Autodesk Inventor part; units mm, degrees
ref_plane "YZ Plane" through (0, 0, 0) normal (1, 0, 0) x (0, 1, 0)
ref_plane "XZ Plane" through (0, 0, 0) normal (0, 1, 0) x (-1, 0, 0)
ref_plane "XY Plane" through (0, 0, 0) normal (0, 0, 1) x (1, 0, 0)
sketch "스케치1" plane through (0, 0, 0) normal (0, 0, 1) x (1, 0, 0)
  line L0 (0, 0) -> (20, 0)
  line L1 (20, 0) -> (20, -20)
  line L2 (20, -20) -> (0, -20)
  line L3 (0, -20) -> (0, 0)
  line L4 (-2, 2) -> (21, 2)
  line L5 (21, 2) -> (21, -22)
  line L6 (21, -22) -> (-2, -22)
  line L7 (-2, -22) -> (-2, 2)
  line L8 (21, 2) -> (21, 5)
  line L9 (21, 5) -> (46, 5)
  line L10 (46, 5) -> (46, -22)
  line L11 (46, -22) -> (21, -22)
  line L12 (22, 3) -> (45, 3)
  line L13 (45, 3) -> (45, -20)
  line L14 (45, -20) -> (22, -20)
  line L15 (22, -20) -> (22, 3)
  line L16 (46, 5) -> (46, 8)
  line L17 (46, 8) -> (74, 8)
  line L18 (74, 8) -> (74, -22)
  line L19 (74, -22) -> (46, -22)
  line L20 (47, 6) -> (73, 6)
  line L21 (73, 6) -> (73, -20)
  line L22 (73, -20) -> (47, -20)
  line L23 (47, -20) -> (47, 6)
  line L24 (74, 8) -> (74, 11)
  line L25 (74, 11) -> (105, 11)
  line L26 (105, 11) -> (105, -22)
  line L27 (105, -22) -> (74, -22)
  line L28 (75, 9) -> (104, 9)
  line L29 (104, 9) -> (104, -20)
  line L30 (104, -20) -> (75, -20)
  line L31 (75, -20) -> (75, 9)
  line L32 (105, 11) -> (105, 14)
  line L33 (105, 14) -> (139, 14)
  line L34 (139, 14) -> (139, -22)
  line L35 (139, -22) -> (105, -22)
  line L36 (106, 12) -> (138, 12)
  line L37 (138, 12) -> (138, -20)
  line L38 (138, -20) -> (106, -20)
  line L39 (106, -20) -> (106, 12)
  line L40 (139, 14) -> (139, 17)
  line L41 (139, 17) -> (177, 17)
  line L42 (177, 17) -> (177, -22)
  line L43 (177, -22) -> (139, -22)
  line L44 (140, 15) -> (175, 15)
  line L45 (175, 15) -> (175, -20)
  line L46 (175, -20) -> (140, -20)
  line L47 (140, -20) -> (140, 15)
  dimension "d0" = 20
  dimension "d1" = 20
  dimension "d2" = 2
  dimension "d3" = 2
  dimension "d4" = 1
  dimension "d5" = 2
  dimension "d6" = 25
  dimension "d7" = 27
  dimension "d8" = 1
  dimension "d9" = 2
  dimension "d10" = 2
  dimension "d11" = 1
  dimension "d12" = 30
  dimension "d13" = 28
  dimension "d14" = 2
  dimension "d15" = 1
  dimension "d16" = 1
  dimension "d17" = 2
  dimension "d18" = 31
  dimension "d19" = 33
  dimension "d20" = 2
  dimension "d21" = 2
  dimension "d22" = 1
  dimension "d23" = 1
  dimension "d24" = 34
  dimension "d25" = 36
  dimension "d26" = 2
  dimension "d27" = 1
  dimension "d28" = 2
  dimension "d29" = 1
  dimension "d30" = 38
  dimension "d31" = 39
  dimension "d32" = 2
  dimension "d33" = 1
  dimension "d34" = 2
  dimension "d35" = 2
extrude "돌출1" add sketch "스케치1" along normal blind 4
sketch "스케치2" plane through (0, 0, 4) normal (0, 0, 1) x (1, 0, 0)
  line L0 (-2, -22) -> (177, -22)
  line L1 (177, -22) -> (177, 17)
  line L2 (177, 17) -> (139, 17)
  line L3 (139, 17) -> (139, 14)
  line L4 (139, 14) -> (105, 14)
  line L5 (105, 14) -> (105, 11)
  line L6 (105, 11) -> (74, 11)
  line L7 (74, 11) -> (74, 8)
  line L8 (74, 8) -> (46, 8)
  line L9 (46, 8) -> (46, 5)
  line L10 (46, 5) -> (21, 5)
  line L11 (21, 5) -> (21, 2)
  line L12 (21, 2) -> (-2, 2)
  line L13 (-2, 2) -> (-2, -22)
  line L14 (22, 3) -> (45, 3)
  line L15 (45, 3) -> (45, -20)
  line L16 (45, -20) -> (22, -20)
  line L17 (22, -20) -> (22, 3)
  line L18 (47, 6) -> (73, 6)
  line L19 (73, 6) -> (73, -20)
  line L20 (73, -20) -> (47, -20)
  line L21 (47, -20) -> (47, 6)
  line L22 (75, 9) -> (104, 9)
  line L23 (104, 9) -> (104, -20)
  line L24 (104, -20) -> (75, -20)
  line L25 (75, -20) -> (75, 9)
  line L26 (106, 12) -> (138, 12)
  line L27 (138, 12) -> (138, -20)
  line L28 (138, -20) -> (106, -20)
  line L29 (106, -20) -> (106, 12)
  line L30 (140, 15) -> (175, 15)
  line L31 (175, 15) -> (175, -20)
  line L32 (175, -20) -> (140, -20)
  line L33 (140, -20) -> (140, 15)
  line L34 (0, 0) -> (20, 0)
  line L35 (20, 0) -> (20, -20)
  line L36 (20, -20) -> (0, -20)
  line L37 (0, -20) -> (0, 0)
extrude "돌출2" add sketch "스케치2" along normal blind 1 contours L13 L12 L11 L10 L9 L8 L7 L6 L5 L4 L3 L2 L1 L0 | L14 L15 L16 L17 | L18 L19 L20 L21 | L22 L23 L24 L25 | L26 L27 L28 L29 | L30 L31 L32 L33 | L34 L35 L36 L37
fillet "모깎기1" radius 2 9 edges at (177, -22, 2.5) (177, 17, 2.5) (139, 17, 2.5) (105, 14, 2.5) (74, 11, 2.5) (46, 8, 2.5) (21, 5, 2.5) (-2, 2, 2.5) (-2, -22, 2.5)
properties part number "d_pocket"
Here's how the part is built. I have some questions about the finished solid (model axes, mm). A direction names the side the tool comes from. Coordinates: 2 decimals unless noted, no trailing zeros. Order: outer loops, then holes, each group sorted by start corner. A loop starts at its lowest first (then second) coordinate and runs counter-clockwise, first axis right, second up.
Item 1: If we section it at A-A, the plane x = 125.5: List the corners of the cut face in (y, z) for me.
Response values:
outline: (-22, 0) - (-20, 0) - (-20, 4) - (12, 4) - (12, 0) - (14, 0) - (14, 5) - (-22, 5) - close
Item 2: I need wall thicknesses on probe 1 along Y at (x, z) = (29.5, 3.35); probe 2 along Y at (x, z) = (81, 1.5); probe 3 along X at (y, z) = (0.5, 2.95). Which ranges of each line are inside material? Lowest first, please.
Response values:
probe 1: y = -22 to -20, 3 to 5
probe 2: y = -22 to -20, 9 to 11
probe 3: x = -1.94 to 22, 45 to 47, 73 to 75, 104 to 106, 138 to 140, 175 to 177
Item 3: If we section it at C-C, the plane z = 0.9: Give the number of separate pieces and of enclosed holes in the cut face, then the cut area to 3 significant figures.
Response values:
separate pieces: 1
enclosed holes: 6
area: 1,090 mm2
Item 4: If we section it at B-B, the plane y = -7: List the corners of the cut face in (x, z) for me.
Response values:
outline: (-2, 0) - (0, 0) - (0, 4) - (20, 4) - (20, 0) - (22, 0) - (22, 4) - (45, 4) - (45, 0) - (47, 0) - (47, 4) - (73, 4) - (73, 0) - (75, 0) - (75, 4) - (104, 4) - (104, 0) - (106, 0) - (106, 4) - (138, 4) - (138, 0) - (140, 0) - (140, 4) - (175, 4) - (175, 0) - (177, 0) - (177, 5) - (-2, 5) - close
Item 5: If we section it at D-D, the plane x = 102.5: List the corners of the cut face in (y, z) for me.
Response values:
outline: (-22, 0) - (-20, 0) - (-20, 4) - (9, 4) - (9, 0) - (11, 0) - (11, 5) - (-22, 5) - close
Item 6: I'm going to push flat-ended pins straight in: pin 1 Ø1.2 at (x, z) = (55, 1) entering from +Y; pin 2 Ø2 at (x, z) = (103, 0.5) entering from +Y; pin 3 Ø6 at (x, y) = (143.5, 2.5) entering from -Z. Where does each tip first touch, or does it pass through?
Response values:
pin 1: stops at y = 8
pin 2: stops at y = 11
pin 3: stops at z = 4
Item 7: Which directions (+Z, -Z, +X, -X, +Y, -Y) give clear straight access to the entire face, cutting with the end or side of a thin tool? Please do faces 4 (the face through (158, -20, 2)), 5 (the face through (10, 2, 2)).
Response values:
face 4: -Z
face 5: +Z, -Z, -X, +Y
Item 8: Thinking about a two-plate mould opening in Y: for faces 1 (the face through (90, 11, 2)), 2 (the face through (122, -20, 2)), 3 (the face through (177, -2, 2)), which applies, pulls with the +Y half, pulls with the -Y half, needs draft (parallel to the pull), parting line crosses it, or undercut?
Response values:
face 1: pulls with the +Y half
face 2: undercut
face 3: needs draft
